```python
from build123d import *

# Parameters (mm, degrees)
BOSS_EXTRUDE1_DEPTH  = 15.696834748
SKETCH6_W            = 13.410834748
SKETCH6_H            = 5.149998248
CUT_EXTRUDE1_DEPTH   = 22.86
BOSS_EXTRUDE7_DEPTH  = 3.175
SKETCH12_R           = 2.8
CUT_EXTRUDE3_DEPTH   = 9.1
SKETCH13_R           = 2.8
CUT_EXTRUDE4_DEPTH   = 9.1
CUT_EXTRUDE6_DEPTH   = 98.762
SKETCH15_R           = 3.175
BOSS_EXTRUDE8_DEPTH  = 19.05
BOSS_EXTRUDE9_DEPTH  = 25.4
BOSS_EXTRUDE10_DEPTH = 25.4
BOSS_EXTRUDE11_DEPTH = 25.4
SKETCH21_W           = 11.024255738
SKETCH21_H           = 18.102082359
BOSS_EXTRUDE12_DEPTH = 6.604


with BuildPart() as part:
    # Sketch1 → Boss-Extrude1 (new body)
    with BuildSketch(Plane.XY):
        Polygon((-68.527338122, 69.932197609), (-69.296818428, 68.086800577), (-71.973324576, 69.203128997), (-77.782900884, 55.270381406), (-82.212980026, 57.11809741), (-84.113890894, 52.559260429), (-79.683811753, 50.711544425), (-80.926887502, 47.730352729), (-87.80424407, 50.598023124), (-73.267575276, 85.460416929), (-27.617891017, 66.425741791), (-42.154559811, 31.563347985), (-57.815709039, 38.093620707), (-56.573548036, 41.072618624), (-52.143468895, 39.22490262), (-50.242558026, 43.783739601), (-54.672637167, 45.631455606), (-48.401372675, 60.671441415), (-51.077878823, 61.787769834), (-50.770086701, 62.525928647), align=None)
    boss_extrude1 = extrude(amount=BOSS_EXTRUDE1_DEPTH)

    # Mirror4: Boss-Extrude1 across plane
    add(boss_extrude1.mirror(Plane(origin=(0, 0, 0), x_dir=(1, 0, 0), z_dir=(0, 0, -1))))

    # Sketch6 → Cut-Extrude1 (cut)
    with BuildSketch(Plane(origin=(-85.89491474, 35.815840233, 0), x_dir=(0, 0, -1), z_dir=(0.9229765876476943, -0.38485610123034036, 0))):
        with Locations((-8.991417374, 33.598495643)):
            Rectangle(SKETCH6_W, SKETCH6_H)
    cut_extrude1 = extrude(amount=-CUT_EXTRUDE1_DEPTH, mode=Mode.SUBTRACT)

    # Mirror5: Cut-Extrude1 across plane
    add(cut_extrude1.mirror(Plane.XY), mode=Mode.SUBTRACT)

    # Sketch8 → Boss-Extrude7 (add, symmetric)
    with BuildSketch(Plane.XY):
        Polygon((-73.267575276, 85.460416929), (-87.80424407, 50.598023124), (-42.154559811, 31.563347985), (-27.617891017, 66.425741791), align=None)
    extrude(amount=BOSS_EXTRUDE7_DEPTH, both=True)

    # Sketch12 → Cut-Extrude3 (cut)
    with BuildSketch(Plane(origin=(19.504696032, 46.776906301, 0), x_dir=(0.9229765876476947, -0.38485610123033953, 0), z_dir=(0.38485610123033953, 0.9229765876476949, 0))):
        with Locations(Location((-81.485896456, 7.968513911, 0), (0, 0, 180))):
            Circle(SKETCH12_R)
        with Locations(Location((-70.563570403, 7.856727715, 0), (0, 0, 180))):
            Circle(SKETCH12_R)
        with Locations(Location((-70.708700217, -6.323512761, 0), (0, 0, 180))):
            Circle(SKETCH12_R)
        with Locations(Location((-81.632170363, -6.323512761, 0), (0, 0, 180))):
            Circle(SKETCH12_R)
    extrude(amount=-CUT_EXTRUDE3_DEPTH, mode=Mode.SUBTRACT)

    # Sketch13 → Cut-Extrude4 (cut)
    with BuildSketch(Plane.XY.offset(15.696834748)):
        with Locations((-45.884678207, 49.584175244)):
            Circle(SKETCH13_R)
        with Locations((-41.590000601, 60.809890325)):
            Circle(SKETCH13_R)
    extrude(amount=-CUT_EXTRUDE4_DEPTH, mode=Mode.SUBTRACT)

    # Sketch14 → Cut-Extrude6 (cut)
    with BuildSketch(Plane.XY.offset(15.696834748)):
        Polygon((-46.640769275, 33.433975157), (-32.104100481, 68.296368962), (-25.409987335, 65.505106084), (-39.946656129, 30.642712279), align=None)
    extrude(amount=-CUT_EXTRUDE6_DEPTH, mode=Mode.SUBTRACT)

    # Sketch15 → Boss-Extrude8 (add)
    with BuildSketch(Plane(origin=(4.968027238, 11.914512496, 0), x_dir=(0.9229765876476949, -0.3848561012303393, 0), z_dir=(-0.3848561012303393, -0.9229765876476949, 0))):
        with Locations(Location((-95.882584307, 0, 0), (0, 0, 180))):
            Circle(SKETCH15_R)
    extrude(amount=BOSS_EXTRUDE8_DEPTH)

    # Sketch17 → Boss-Extrude9 (add)
    with BuildSketch(Plane.XY.offset(15.696834748)):
        Polygon((-51.077878823, 61.787769834), (-48.401372675, 60.671441415), (-43.173444366, 72.911983906), (-73.267575276, 85.460416929), (-78.850681144, 72.070799392), (-71.973324576, 69.203128997), (-69.296818428, 68.086800577), (-68.527338122, 69.932197609), (-50.770086701, 62.525928647), align=None)
        Polygon((-84.113890894, 52.559260429), (-82.212980026, 57.11809741), (-77.782900884, 55.270381406), (-73.955332823, 64.449801187), (-80.832689391, 67.317471582), (-87.80424407, 50.598023124), (-80.926887502, 47.730352729), (-79.683811753, 50.711544425), align=None)
        Polygon((-43.497872754, 40.971389524), (-50.242558026, 43.783739601), (-52.143468895, 39.22490262), (-56.573548036, 41.072618624), (-57.815709039, 38.093620707), (-46.640769275, 33.433975157), align=None)
    boss_extrude9 = extrude(amount=BOSS_EXTRUDE9_DEPTH)

    # Sketch18 → Boss-Extrude10 (add)
    with BuildSketch(Plane.XY.offset(3.175)):
        Polygon((-79.683811753, 50.711544425), (-80.926887502, 47.730352729), (-57.815709039, 38.093620707), (-56.573548036, 41.072618624), (-52.143468895, 39.22490262), (-50.242558026, 43.783739601), (-54.672637167, 45.631455606), (-48.401372675, 60.671441415), (-51.077878823, 61.787769834), (-50.770086701, 62.525928647), (-68.527338122, 69.932197609), (-69.296818428, 68.086800577), (-71.973324576, 69.203128997), (-78.850681144, 72.070799392), (-80.832689391, 67.317471582), (-73.955332823, 64.449801187), (-77.782900884, 55.270381406), (-82.212980026, 57.11809741), (-84.113890894, 52.559260429), align=None)
    boss_extrude10 = extrude(amount=BOSS_EXTRUDE10_DEPTH)

    # Mirror6: Boss-Extrude9, Boss-Extrude10 across plane
    add(boss_extrude9.mirror(Plane.XY))
    add(boss_extrude10.mirror(Plane.XY))

    # Sketch19 → Boss-Extrude11 (add)
    with BuildSketch(Plane(origin=(0, 0, -15.696834748), x_dir=(-1, 0, 0), z_dir=(0, 0, -1))):
        Polygon((43.497872754, 40.971389524), (50.242558026, 43.783739601), (54.672637167, 45.631455606), (48.401372675, 60.671441415), (43.173444366, 72.911983906), (32.104100481, 68.296368962), align=None)
    extrude(amount=BOSS_EXTRUDE11_DEPTH)

    # Sketch21 → Boss-Extrude12 (add)
    with BuildSketch(Plane(origin=(4.968027238, 11.914512496, 0), x_dir=(0.9229765876476949, -0.3848561012303393, 0), z_dir=(-0.3848561012303393, -0.9229765876476949, 0))):
        with Locations((-95.002091614, -1.001456214)):
            Rectangle(SKETCH21_W, SKETCH21_H)
    extrude(amount=BOSS_EXTRUDE12_DEPTH)


solid = part.part
```
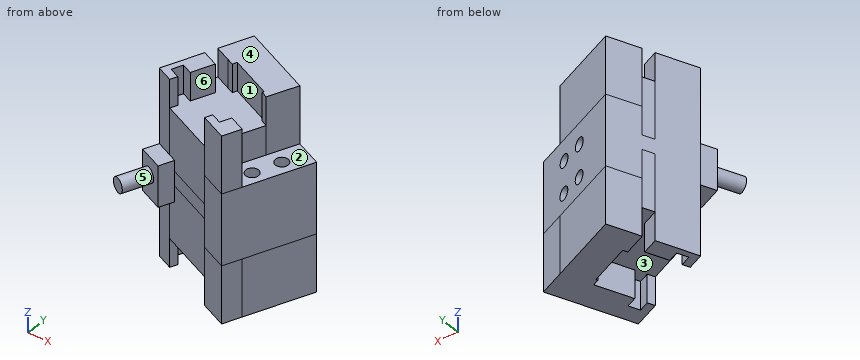
Source: CAD feature listing. Evaluate the final solid. Frame: model axes, mm. Face numbers are marked on the shaded views. A direction names the side the tool comes from. Coordinates: 2 decimals unless noted, no trailing zeros. Order: outer loops, then holes, each group sorted by start corner. A loop starts at its lowest first (then second) coordinate and runs counter-clockwise, first axis right, second up. Notation, with made-up numbers: M 17.5,53 L 54.5,53 A16 ccw 54.5,76 Z; hole C 31,-20.75 d3. An arc over 180 degrees is marked long. Write each question's results on one line, items separated by ' | '. Start each with the question number.
1) Section query D-D (z = 27.5). Return the cut outline in (x, y), plus the area to 3 significant figures.
2) Contact query for flat-ended pins moving along their axis: pin 1 Ø3 at (x, y) = (-43, 60) entering from +Z; pin 2 Ø12 at (x, y) = (-66, 40.5) entering from -Z (3 decimals); pin 3 Ø10 at (x, z) = (-41.5, -2) entering from +Y. Output: stop coordinate, or through.
3) Section query A-A (z = -21.5). Return the cut outline in (x, y), plus the area to 3 significant figures.
4) Draft query along Y for the marked faces 4, 5 and 6. Return one class per face: released by +Y, released by -Y, zero draft, split by the parting line, or undercut.
5) Section query C-C (z = 11.5). Return the cut outline in (x, y).
6) Section query B-B (x = -41.59). Return the cut outline in (y, z), plus the area to 3 significant figures.
7) Line query: line 1 (Z direction, x = -57, y = 77); line 2 (Z direction, x = -80.5, y = 53.5) (3 decimals); line 3 (Y direction, x = -52, z = -32.5). Output: solid intervals per line, ascending. Write a range as from..to.
8) Access query for the marked faces 1, 2 and 3. Directions: +Z, -Z, +X, -X, +Y, -Y. A direction counts if a zero-diameter tool reaches every point of the face in a straight line with its end or side. Return the directions, or none.
Answers:
1) outline: M -87.8,50.6 L -46.64,33.43 L -43.5,40.97 L -50.24,43.78 L -54.67,45.63 L -48.4,60.67 L -43.17,72.91 L -73.27,85.46 Z | area: 1,330 mm^2
2) pin 1: stops at z = 15.7 | pin 2: stops at z = -28.575 | pin 3: stops at y = 74.3
3) outline: M -87.8,50.6 L -46.64,33.43 L -32.1,68.3 L -73.27,85.46 Z | area: 1,680 mm^2
4) face 4: zero draft | face 5: undercut | face 6: released by -Y
5) outline: M -87.8,50.6 L -46.64,33.43 L -32.1,68.3 L -73.27,85.46 Z; hole C -45.88,49.58 d5.6; hole C -41.59,60.81 d5.6
6) outline: M 45.55,-41.1 L 72.25,-41.1 L 72.25,15.7 L 63.61,15.7 L 63.61,6.6 L 58.01,6.6 L 58.01,15.7 L 45.55,15.7 Z | area: 1,470 mm^2
7) line 1: z = -41.1..-10.66, -5.27..3.59, 9.06..41.1 | line 2: z = -28.575..28.575 | line 3: y = 35.67..39.57, 44.52..52.04, 63.04..76.59
8) face 1: +Z | face 2: +Z, +X | face 3: -Z
